Model file for the job. Use its own axes, mm. Round coordinates to 2 decimals unless told otherwise and drop trailing zeros. Order: outer loops, then holes, each group sorted by start corner. A loop starts at its lowest first (then second) coordinate and runs counter-clockwise, first axis right, second up. Notation, with made-up numbers: (-5, -38) - (31, -38) arc R22 ccw to (31, -5) - close; hole circle Ø3 at (23.25, 5.25). An arc over 180 degrees is marked (long way). Put each result on its own line as item: value. Start each with the question number.
Item 1: Saw through at A-A on y = 0. List the corners of the cut face in (x, z) (3 decimals), plus the area to 3 significant figures.
Item 2: Saw through at D-D on x = 8.25. List the corners of the cut face in (y, z) (3 decimals).
Item 3: Saw through at B-B on z = 0. List the corners of the cut face in (x, y) (3 decimals), plus the area to 3 significant figures.
Item 4: Probe probe 1 along X at (y, z) = (-2, 0.25) (3 decimals); probe 2 along Z at (x, y) = (0, 2); probe 3 along Z at (x, y) = (-1, 1.5). List the from-to ranges inside material, lowest first.
Item 5: Mould opens along Z. For faces 1 (the face through (-2.09, 0.07, -2.47)), 2 (the face through (0.12, -0.21, -4.81)), 3 (the face through (-9.525, 0, 0)) say: pulls with the +Z half, pulls with the -Z half, needs draft (parallel to the pull), parting line crosses it, or undercut.
Item 6: Pin check, flat tips, straight feed: pin 1 Ø1.5 at (x, z) = (2, 2.5) entering from -Y; pin 2 Ø2 at (x, z) = (-4.5, -3.5) entering from -Y. Stop position of each tip, or through.
Item 7: Saw through at C-C on x = 0. List the corners of the cut face in (y, z) (1 decimal).
```python
from build123d import *

# Parameters (mm, degrees)
SKETCH1_R           = 4.815
BOSS_EXTRUDE1_DEPTH = 9.525
CHAMFER1_SIZE       = 0.76
SKETCH2_R           = 3.43
CUT_EXTRUDE1_DEPTH  = 95.25


with BuildPart() as part:
    # Sketch1 → Boss-Extrude1 (new, symmetric)
    with BuildSketch(Plane(origin=(0, 0, 0), x_dir=(0, 0, -1), z_dir=(1, 0, 0))):
        with Locations(Location((0, 0, 0), (0, 0, 180))):
            Circle(SKETCH1_R)
    extrude(amount=BOSS_EXTRUDE1_DEPTH, both=True)

    # Chamfer1
    chamfer1_edges = [part.edges().sort_by_distance(p)[0] for p in [
        (-9.525, 0, -4.815),
        (9.525, 0, -4.815),
    ]]
    chamfer(chamfer1_edges, length=CHAMFER1_SIZE)

    # Sketch2 → Cut-Extrude1 (cut, symmetric)
    with BuildSketch(Plane(origin=(0, 0, 0), x_dir=(1, 0, 0), z_dir=(0, 1, 0))):
        with Locations(Location((0, -0.25, 0), (0, 0, 270))):
            Circle(SKETCH2_R)
    extrude(amount=CUT_EXTRUDE1_DEPTH, both=True, mode=Mode.SUBTRACT)


solid = part.part
```
Results found:
1. outline: (-9.525, -4.055) - (-8.765, -4.815) - (8.765, -4.815) - (9.525, -4.055) - (9.525, 4.055) - (8.765, 4.815) - (-8.765, 4.815) - (-9.525, 4.055) - close; hole circle Ø6.86 at (0, 0.25)
1. area: 145 mm²
2. outline: circle Ø9.63 at (0, 0)
3. outline: (-9.525, -4.055) - (-8.765, -4.815) - (-3.421, -4.815) - (-3.421, 4.815) - (-8.765, 4.815) - (-9.525, 4.055) - close; (3.421, -4.815) - (8.765, -4.815) - (9.525, -4.055) - (9.525, 4.055) - (8.765, 4.815) - (3.421, 4.815) - close
3. area: 116 mm²
4. probe 1: x = -9.525 to -3.43, 3.43 to 9.525
4. probe 2: z = -4.38 to -3.18, 3.68 to 4.38
4. probe 3: z = -4.58 to -3.03, 3.53 to 4.58
5. face 1: undercut
5. face 2: parting line crosses it
5. face 3: needs draft
6. pin 1: stops at y = -4.22
6. pin 2: stops at y = -4.12
7. outline: (-3.6, -3.2) arc R4.8 ccw to (3.6, -3.2) - close; (-3.1, 3.7) - (3.1, 3.7) arc R4.8 ccw to start
